Here's how the part is built. I have some questions about the finished solid (model axes, mm). Face numbers are marked on the shaded views. A direction names the side the tool comes from. Coordinates: 2 decimals unless noted, no trailing zeros. Write each loop counter-clockwise with the first axis right and the second up, starting at its lowest first coordinate (ties: lowest second). Pieces come first, ordered by that corner, then holes. Notation, with made-up numbers: M 5,47 L 36,47 A14 ccw 36,56 Z; hole C -35,-21.5 d4. An arc over 180 degrees is marked long. Write each question's results on one line, items separated by ' | '. Start each with the question number.
from build123d import *

# Parameters (mm, degrees)
F0_W          = 100.2182774246
F0_H          = 82.0081606507
F3_DEPTH      = 40
F4_D          = 10
F4_DEPTH      = 54.9592019448
F5_D          = 10
F1_W          = 44.1022608429
F1_H          = 32.8041445464
F6_DEPTH      = 60.3
F6_DEPTH_BACK = 51.5
F7_W          = 92.5000049174
F7_H          = 76.2500017881
F8_DEPTH      = 52.4
F8_DEPTH_BACK = 25


with BuildPart() as f3:
    # F0 (on Top) → F3 (new body)
    with BuildSketch(Plane.XY):
        with Locations((4.8490632325, 5.9297867119)):
            Rectangle(F0_W, F0_H)
    extrude(amount=F3_DEPTH)

    # F4 (through all, one way)
    with BuildSketch(Plane(origin=(0, 0, 0), x_dir=(0, 1, 0), z_dir=(-1, 0, 0))):
        with Locations((4.6449177898, -24.9448493123)):
            Circle(F4_D / 2)
    extrude(amount=-F4_DEPTH, mode=Mode.SUBTRACT)

    # F5 (through all)
    with Locations(Plane.YZ):
        with Locations((4.6449177898, 24.9448493123)):
            Hole(F5_D / 2)

    # F1 (on Front) → F6 (cut, two sides)
    with BuildSketch(Plane.XZ) as f6_sk:
        with Locations((7.1431370452, 36.986050196)):
            Rectangle(F1_W, F1_H)
    extrude(amount=-F6_DEPTH, mode=Mode.SUBTRACT)
    extrude(f6_sk.sketch, amount=F6_DEPTH_BACK, mode=Mode.SUBTRACT)

    # F7 (on Top) → F8 (cut, two sides)
    with BuildSketch(Plane.XY) as f8_sk:
        with Locations((5.0000008196, 5.7500004768)):
            Rectangle(F7_W, F7_H)
    extrude(amount=F8_DEPTH, mode=Mode.SUBTRACT)
    extrude(f8_sk.sketch, amount=-F8_DEPTH_BACK, mode=Mode.SUBTRACT)


solid = f3.part
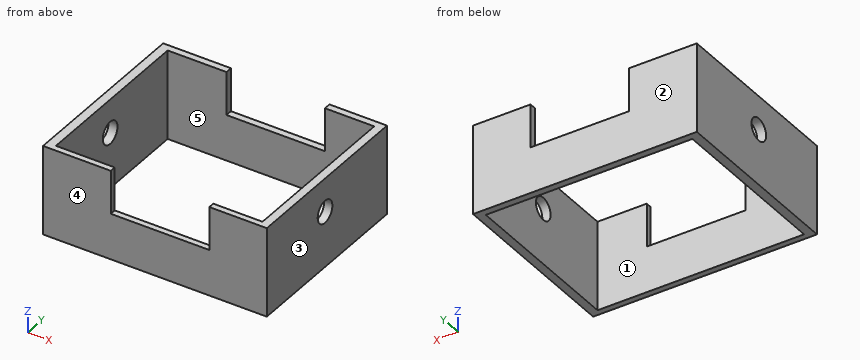
1) For pin 1 Ø2.5 at (x, y) = (4.5, 46) entering from +Z, with a flat end and sliding along its axis, tell me the tip position at first contact or that it passes through.
2) I want a section at A-A, the plane x = 48. Write out the boundary of the cut face in (y, z) (3 decimals).
3) I want a section at D-D, the plane z = 35. Write out the boundary of the cut face in (x, y) (3 decimals).
4) I want a section at B-B, the plane z = 13. Write out the boundary of the cut face in (x, y) (3 decimals), then the cut area to 3 significant figures.
5) For the marked faces 1 and 2, which set-ups out of +Z, -Z, +X, -X, +Y, -Y let a thin tool reach every point of the face, with its end or its side?
6) I want a section at C-C, the plane y = 29.5. Write out the boundary of the cut face in (x, z).
7) Please list where these lines run through material, in increasing order: line 1 (X direction, y = -26, z = 34); line 2 (Y direction, x = -41, z = 32) (3 decimals). Write a range as [from, to].
8) We'd pull the mould along Y, two halves only. Please class the marked faces 3, 4 and 5: pulls with the +Y half, pulls with the -Y half, needs draft (parallel to the pull), parting line crosses it, or undercut.
Output:
1) pin 1: stops at z = 20.58
2) outline: M -35.074,0 L -32.375,0 L -32.375,40 L -35.074,40 Z; M 43.875,0 L 46.934,0 L 46.934,40 L 43.875,40 Z
3) outline: M -45.26,-35.074 L -14.908,-35.074 L -14.908,-32.375 L -41.25,-32.375 L -41.25,43.875 L -14.908,43.875 L -14.908,46.934 L -45.26,46.934 Z; M 29.194,-35.074 L 54.958,-35.074 L 54.958,46.934 L 29.194,46.934 L 29.194,43.875 L 51.25,43.875 L 51.25,-32.375 L 29.194,-32.375 Z
4) outline: M -45.26,-35.074 L 54.958,-35.074 L 54.958,46.934 L -45.26,46.934 Z; hole M -41.25,-32.375 L 51.25,-32.375 L 51.25,43.875 L -41.25,43.875 Z | area: 1,170 mm2
5) face 1: +Z, -Z | face 2: +Z, -Z, +X, -X, +Y
6) outline: M -45.26,0 L -41.25,0 L -41.25,40 L -45.26,40 Z; M 51.25,0 L 54.96,0 L 54.96,40 L 51.25,40 Z
7) line 1: x = [-45.26, -41.25], [51.25, 54.96] | line 2: y = [-35.074, -32.375], [43.875, 46.934]
8) face 3: needs draft | face 4: pulls with the -Y half | face 5: undercut
